Autodesk Inventor part; units mm, degrees
ref_plane "YZ Plane" through (0, 0, 0) normal (1, 0, 0) x (0, 1, 0)
ref_plane "XZ Plane" through (0, 0, 0) normal (0, 1, 0) x (-1, 0, 0)
ref_plane "XY Plane" through (0, 0, 0) normal (0, 0, 1) x (1, 0, 0)
sketch "Esboço1" plane through (0, 0, 0) normal (0, 1, 0) x (-1, 0, 0)
  line L0 (0, 0) -> (60, 0)
  line L1 (60, 0) -> (60, -12)
  line L2 (60, -12) -> (60, -19)
  line L3 (60, -19) -> (60, -53)
  line L4 (60, -53) -> (60, -60)
  line L5 (60, -60) -> (60, -72)
  line L6 (60, -72) -> (0, -72)
  line L7 (0, -72) -> (0, 0)
  line L8 (0, 0) -> (19, 0)
  line L9 (60, 0) -> (30, 0)
  circle A0 centre (45, -16) radius 3.5
  circle A1 centre (45, -56) radius 3.5
  circle A2 centre (9.5, -16) radius 3.5
  circle A3 centre (9.5, -56) radius 3.5
  dimension "d0" = 60
  dimension "d1" = 12
  dimension "d2" = 7
  dimension "d3" = 34
  dimension "d4" = 7
  dimension "d5" = 12
  dimension "d6" = 72
  dimension "d7" = 19
  dimension "d12" = 30
  dimension "d23" = 7
  dimension "d24" = 7
  dimension "d25" = 7
  dimension "d26" = 7
extrude "Extrusão2" add sketch "Esboço1" along normal blind 1.2
fillet "Arredondamento2" radius 2 4 edges at (-60, 0.6, 0) (-60, 0.6, -72) (0, 0.6, 0) (0, 0.6, -72)
sketch "Esboço2" plane through (0, 1.2, 0) normal (0, 1, 0) x (1, 0, 0)
  circle A0 centre (-45, 56) radius 3.5
  line L0 (-45, 56) -> (-30, 56)
  line L1 (-30, 56) -> (-20, 56)
  line L2 (0, 2) -> (0, 70)
  circle A1 centre (-9.5, 16) radius 3.5
  circle A2 centre (-9.5, 36) radius 1.75
  point P0 (0, 0)
  dimension "d30" = 15
  dimension "d31" = 10
extrude "Extrusão5" cut sketch "Esboço2" against normal blind 10 contours A2
properties part number "chapa-fixação-caixa" material "Aço galvanizado"
CAD build for the part. Positions are in the model's coordinates, mm. Coordinates: 2 decimals unless noted, no trailing zeros. Write each loop counter-clockwise with the first axis right and the second up, starting at its lowest first coordinate (ties: lowest second). Pieces come first, ordered by that corner, then holes. Notation, with made-up numbers: (73.5, 59.25) -> (94.5, 59.25) arc R26 ccw to (94.5, 92.25) -> close; hole circle Ø5 at (67.5, 12.5). An arc over 180 degrees is marked (long way). Return JSON: item names as keys, results as strings. Group by question number.
Q1. Cut at A-A, the plane z = -36. Give the cut face in (x, y).
Q2. Cut at C-C, the plane z = -16. Give the cut face in (x, y), then the cut area to 3 significant figures.
Q3. Cut at B-B, the plane x = -45. Give the cut face in (y, z).
Q4. Drill centre lines: line 1 (Z direction, x = -45, y = 0.3); line 2 (Z direction, x = -9.5, y = 0.7); line 3 (X direction, y = 0.95, z = -36). Where is each one in solid material? Low to high.
Q5. Pull direction X, two halves, no side cores. Call faces 1 (the face through (-6, 1, -56)), 2 (the face through (-30, 1.2, -35)), 3 (the face through (-0.57, 0.61, -71.4)): released by +X, released by -X, zero draft, split by the parting line, or undercut.
Q6. Cut at D-D, the plane y = 0.75. Give the cut face in (x, z).
Returned:
{
 "1": {"outline": "(-60, 0) -> (-11.25, 0) -> (-11.25, 1.2) -> (-60, 1.2) -> close; (-7.75, 0) -> (0, 0) -> (0, 1.2) -> (-7.75, 1.2) -> close"},
 "2": {"outline": "(-60, 0) -> (-48.5, 0) -> (-48.5, 1.2) -> (-60, 1.2) -> close; (-41.5, 0) -> (-13, 0) -> (-13, 1.2) -> (-41.5, 1.2) -> close; (-6, 0) -> (0, 0) -> (0, 1.2) -> (-6, 1.2) -> close", "area": "55.2 mm2"},
 "3": {"outline": "(0, -72) -> (1.2, -72) -> (1.2, -59.5) -> (0, -59.5) -> close; (0, -52.5) -> (1.2, -52.5) -> (1.2, -19.5) -> (0, -19.5) -> close; (0, -12.5) -> (1.2, -12.5) -> (1.2, 0) -> (0, 0) -> close"},
 "4": {"line 1": "z = -72 to -59.5, -52.5 to -19.5, -12.5 to 0", "line 2": "z = -72 to -59.5, -52.5 to -37.75, -34.25 to -19.5, -12.5 to 0", "line 3": "x = -60 to -11.25, -7.75 to 0"},
 "5": {"face 1": "undercut", "face 2": "zero draft", "face 3": "released by +X"},
 "6": {"outline": "(-60, -70) arc R2 ccw to (-58, -72) -> (-2, -72) arc R2 ccw to (0, -70) -> (0, -2) arc R2 ccw to (-2, 0) -> (-58, 0) arc R2 ccw to (-60, -2) -> close; hole circle Ø7 at (-45, -56); hole circle Ø7 at (-45, -16); hole circle Ø7 at (-9.5, -56); hole circle Ø7 at (-9.5, -16); hole circle Ø3.5 at (-9.5, -36)"}
}
